Autodesk Inventor part; units mm, degrees
ref_plane "YZ Plane" through (0, 0, 0) normal (1, 0, 0) x (0, 1, 0)
ref_plane "XZ Plane" through (0, 0, 0) normal (0, 1, 0) x (-1, 0, 0)
ref_plane "XY Plane" through (0, 0, 0) normal (0, 0, 1) x (1, 0, 0)
sketch "Sketch1" plane through (0, 0, 0) normal (0, 1, 0) x (-1, 0, 0)
  line L0 (-344.259, 333.63) -> (-369.659, 333.63)
  line L1 (-369.659, 333.63) -> (-369.659, 28.83)
  line L2 (-369.659, 28.83) -> (-344.259, 28.83)
  line L3 (-344.259, 28.83) -> (-344.259, 333.63)
  point P0 (0, 0)
  dimension "d0" = 25.4
  dimension "d1" = 304.8
extrude "Extrusion1" add sketch "Sketch1" along normal blind 11.938
sketch "Sketch2" plane through (0, 11.938, 0) normal (0, 1, 0) x (1, 0, 0)
  line L0 (369.659, -28.83) -> (344.259, -28.83)
  line L1 (356.959, -28.83) -> (356.959, -333.63) construction
  circle A0 centre (356.959, -41.53) radius 2.3813
  circle A1 centre (356.959, -54.23) radius 2.3813
  circle A2 centre (356.959, -66.93) radius 2.3813
  circle A3 centre (356.959, -79.63) radius 2.3813
  circle A4 centre (356.959, -92.33) radius 2.3813
  circle A5 centre (356.959, -105.03) radius 2.3813
  circle A6 centre (356.959, -117.73) radius 2.3813
  circle A7 centre (356.959, -130.43) radius 2.3813
  circle A8 centre (356.959, -143.13) radius 2.3813
  circle A9 centre (356.959, -155.83) radius 2.3813
  circle A10 centre (356.959, -168.53) radius 2.3813
  circle A11 centre (356.959, -181.23) radius 2.3813
  circle A12 centre (356.959, -193.93) radius 2.3813
  circle A13 centre (356.959, -206.63) radius 2.3813
  circle A14 centre (356.959, -219.33) radius 2.3813
  circle A15 centre (356.959, -232.03) radius 2.3813
  circle A16 centre (356.959, -244.73) radius 2.3813
  circle A17 centre (356.959, -257.43) radius 2.3813
  circle A18 centre (356.959, -270.13) radius 2.3813
  circle A19 centre (356.959, -282.83) radius 2.3813
  circle A20 centre (356.959, -295.53) radius 2.3813
  circle A21 centre (356.959, -308.23) radius 2.3813
  circle A22 centre (356.959, -320.93) radius 2.3813
  point P0 (0, 0)
  dimension "d20" = 4.7625
  dimension "d21" = 12.7
  dimension "d24" = 12.7
hole "Hole1" at (356.959, 11.938, 41.53) at (356.959, 11.938, 54.23) at (356.959, 11.938, 66.93) at (356.959, 11.938, 79.63) at (356.959, 11.938, 92.33) at (356.959, 11.938, 105.03) at (356.959, 11.938, 117.73) at (356.959, 11.938, 130.43) at (356.959, 11.938, 143.13) at (356.959, 11.938, 155.83) at (356.959, 11.938, 168.53) at (356.959, 11.938, 181.23) at (356.959, 11.938, 193.93) at (356.959, 11.938, 206.63) at (356.959, 11.938, 219.33) at (356.959, 11.938, 232.03) at (356.959, 11.938, 244.73) at (356.959, 11.938, 257.43) at (356.959, 11.938, 270.13) at (356.959, 11.938, 282.83) at (356.959, 11.938, 295.53) at (356.959, 11.938, 308.23) at (356.959, 11.938, 320.93) direction (0, -1, 0) diameter 4.7625 end through all
properties part number "linkage"
Could you check a few things on this model? Use its own coordinates, in mm. Coordinates: 2 decimals unless noted, no trailing zeros. One line per question, with ' | ' between items.
Q1. Thinking about a two-plate mould opening in X: for faces 1 (the face through (354.6, 5.9, 257.1)), 2 (the face through (354.6, 5.9, 104.7)), 3 (the face through (344.259, 6, 179)), which applies, pulls with the +X half, pulls with the -X half, needs draft (parallel to the pull), parting line crosses it, or undercut?
Return value:
face 1: undercut | face 2: undercut | face 3: pulls with the -X half
Q2. Imagine slicing it at A-A on y = 9.5. State how many separate pieces and enclosed holes the cut face has, and give its area (3 significant figures).
Return value:
separate pieces: 1 | enclosed holes: 23 | area: 7,330 mm²
Q3. I'm going to push a flat-ended pin straight in: P1, Ø12, axis at x = 366.5, z = 190, coming from the -Y side. Where does the tip first touch, or does it pass through?
Return value:
P1: y = 0
Q4. If I drill on L1, parallel to X at y = 3, z = 244.73; L2, parallel to X at y = 9.5, z = 195, over which ranges is the centre line in solid material (lowest first)?
Return value:
L1: 344.26 to 354.58, 359.34 to 369.66 | L2: 344.26 to 354.83, 359.09 to 369.66
